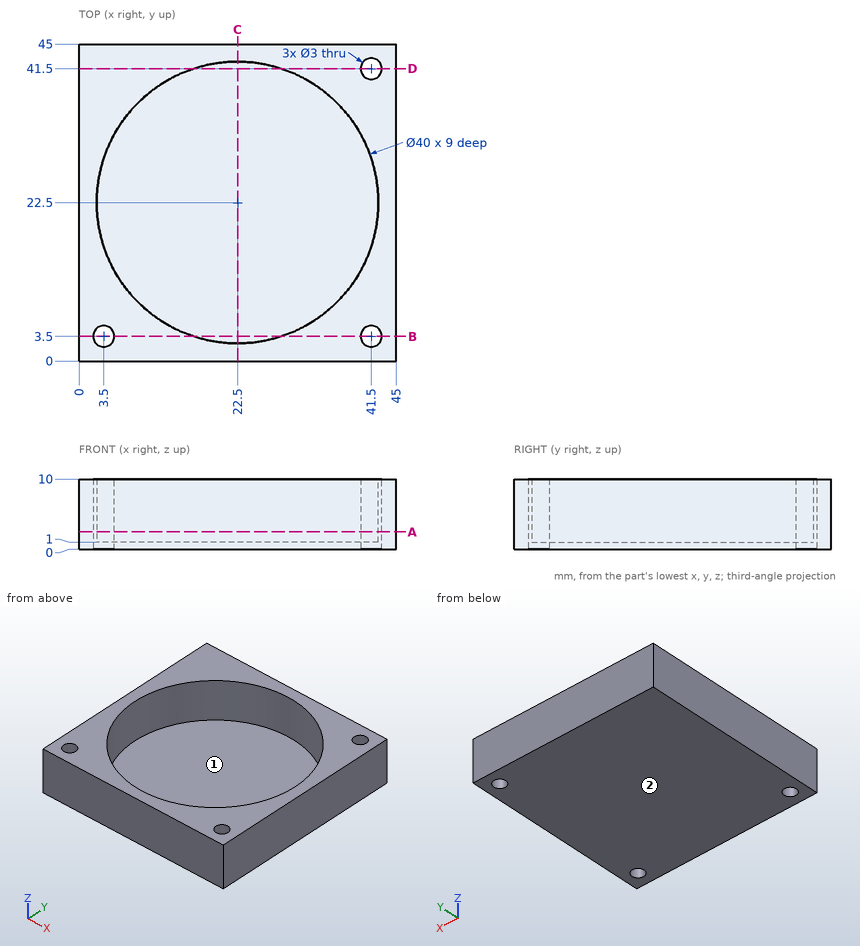
Job drawing, mm, ordinate dimensions from the low corner. One solid piece. A direction names the side the tool comes from. Give positions to 0.01 mm unless a question says otherwise; leave off trailing zeros. Order: outer loops, then holes, each group sorted by start corner. A loop starts at its lowest first (then second) coordinate and runs counter-clockwise, first axis right, second up. Notation, with made-up numbers: (68, -29) - (108, -29) arc R16 ccw to (108, -3) - close; hole circle Ø11 at (-14.5, -9). An arc over 180 degrees is marked (long way). One line per question, with ' | ' between items.
1. Band-saw the part on D-D on y = 41.5. List the corners of the cut face in (x, z) (3 decimals).
Filled in:
outline: (0, 0) - (40, 0) - (40, 10) - (28.745, 10) - (28.745, 1) - (16.255, 1) - (16.255, 10) - (0, 10) - close; (43, 0) - (45, 0) - (45, 10) - (43, 10) - close
2. Band-saw the part on C-C on x = 22.5. List the corners of the cut face in (y, z).
Filled in:
outline: (0, 0) - (45, 0) - (45, 10) - (42.5, 10) - (42.5, 1) - (2.5, 1) - (2.5, 10) - (0, 10) - close
3. Band-saw the part on A-A on z = 2.5. List the corners of the cut face in (x, y).
Filled in:
outline: (0, 0) - (45, 0) - (45, 45) - (0, 45) - close; hole circle Ø3 at (3.5, 3.5); hole circle Ø40 at (22.5, 22.5); hole circle Ø3 at (41.5, 3.5); hole circle Ø3 at (41.5, 41.5)
4. Which spindle directions (+Z, -Z, +X, -X, +Y, -Y) get a long thin tool onto all of the face, cutting with end or side? Do the marked faces 1 and 2. Say none if no direction does.
Filled in:
face 1: +Z | face 2: -Z, +X, -X, +Y, -Y
5. Band-saw the part on B-B on y = 3.5. List the corners of the cut face in (x, z) (3 decimals).
Filled in:
outline: (0, 0) - (2, 0) - (2, 10) - (0, 10) - close; (5, 0) - (40, 0) - (40, 10) - (28.745, 10) - (28.745, 1) - (16.255, 1) - (16.255, 10) - (5, 10) - close; (43, 0) - (45, 0) - (45, 10) - (43, 10) - close
6. Drill centre lines: probe 1 along Y at (x, z) = (22.5, 8); probe 2 along Y at (x, z) = (11.5, 5.5). Where is each one in solid material? Low to high.
Filled in:
probe 1: 0 to 2.5, 42.5 to 45 | probe 2: 0 to 5.8, 39.2 to 45
7. Drop a flat-ended pin along its axis: P1, Ø2.5, axis at x = 3.5, y = 3.5, coming from the +Z side. Give the stop position or say it passes through.
Filled in:
P1: through
